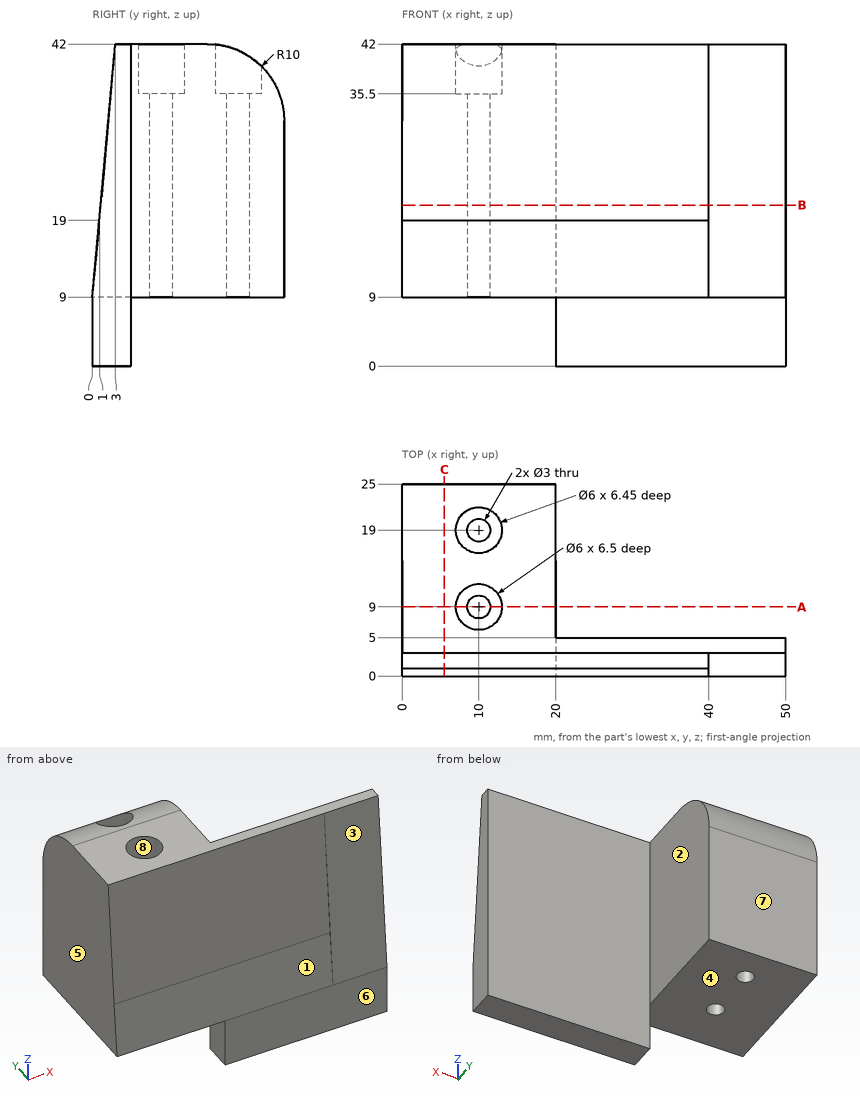
Design review of the part shown in the three views and the two pictorial views. Dimensions are in mm from the part's minimum x, y and z. A direction names the side the tool comes from. Give positions to 0.01 mm unless a question says otherwise; leave off trailing zeros. Write each loop counter-clockwise with the first axis right and the second up, starting at its lowest first coordinate (ties: lowest second). Pieces come first, ordered by that corner, then holes. Notation, with made-up numbers: M 58,-6.5 L 116,-6.5 A17 cw 116,22.5 Z; hole C 3.5,88 d4. An arc over 180 degrees is marked long. Answer as CSV lines item,"result".
1. Wall thickness on line 1 (Y direction, x = 10, z = 22.75); line 2 (Y direction, x = 10, z = 30); line 3 (Z direction, x = 17, y = 7.75): over which ranges is each line inside the solid? List them lowest first.
Findings:
line 1,"y = 1.33 to 7.5, 10.5 to 17.5, 20.5 to 25"
line 2,"y = 1.96 to 7.5, 10.5 to 17.5, 20.5 to 25"
line 3,"z = 9 to 42"
2. Consider section A-A, the plane y = 9. Write out the cut boundary in (x, z).
Findings:
outline,"M 0,9 L 8.5,9 L 8.5,35.5 L 7,35.5 L 7,42 L 0,42 Z; M 11.5,9 L 20,9 L 20,42 L 13,42 L 13,35.5 L 11.5,35.5 Z"
3. For pin 1 (8 mm diameter, centred on x = 23.5, z = 17, fed in from -Y); pin 2 (3 mm diameter, centred on x = 11, y = 8, fed in from +Z); pin 3 (7 mm diameter, centred on x = 10, y = 9, fed in from -Z), all flat-tipped, find the tip position at first contact; note any pin that passes through.
Findings:
pin 1,"stops at y = 0.4"
pin 2,"stops at z = 35.5"
pin 3,"stops at z = 9"
4. Consider section B-B, the plane z = 21. Write out the cut boundary in (x, y).
Findings:
outline,"M 0,1.17 L 40,1.17 L 40,1.09 L 50,1.09 L 50,5 L 20,5 L 20,25 L 0,25 Z; hole C 10,9 d3; hole C 10,19 d3"
5. Consider section C-C, the plane x = 5.5. Write out the cut boundary in (y, z).
Findings:
outline,"M 0,9 L 25,9 L 25,32 A10 ccw 15,42 L 3,42 L 1,19 Z"
6. Draft analysis for pull direction Y (two halves, no side actions). For the marked faces 6, 7 and 8, state which applies: +Y half, -Y half, draft (parallel to the pull), parting line (faces both ways), or undercut.
Findings:
face 6,"-Y half"
face 7,"+Y half"
face 8,"undercut"
7. For the marked faces 1, 2, 3, 4 and 5, list the 3-axis set-ups (+Z, -Z, +X, -X, +Y, -Y) from which the entire face can be reached by the end or side of a thin tool; tool diameter is ignored.
Findings:
face 1,"+Z, -X, -Y"
face 2,"+Z, -Z, +X, +Y"
face 3,"+Z, +X, -X, -Y"
face 4,"-Z, -X, +Y, -Y"
face 5,"+Z, -Z, -X, +Y, -Y"
